Here's how the part is built. I have some questions about the finished solid (model axes, mm). Give positions to 0.01 mm unless a question says otherwise; leave off trailing zeros. Write each loop counter-clockwise with the first axis right and the second up, starting at its lowest first coordinate (ties: lowest second). Pieces come first, ordered by that corner, then holes. Notation, with made-up numbers: (49.5, 33) - (93.5, 33) arc R6 ccw to (93.5, 42) - close; hole circle Ø2 at (-26, -9.5). An arc over 180 degrees is marked (long way). Use a Markdown table: item, result.
Autodesk Inventor part; units mm, degrees
ref_plane "YZ Plane" through (0, 0, 0) normal (1, 0, 0) x (0, 1, 0)
ref_plane "XZ Plane" through (0, 0, 0) normal (0, 1, 0) x (-1, 0, 0)
ref_plane "XY Plane" through (0, 0, 0) normal (0, 0, 1) x (1, 0, 0)
sketch "スケッチ1" plane through (0, 0, 0) normal (0, 0, 1) x (1, 0, 0)
  circle A0 centre (104.0735, 2) radius 6.025
  arc A1 (100.4168, -2.7885) -> (70.6822, 5.0468) centre (76.1402, -34.5791) ccw
  line L0 (69.7806, -5) -> (104.0735, 2) construction
  circle A2 centre (69.7806, -5) radius 5 construction
  arc A3 (102.7574, -3.8795) -> (72.4739, -9.2126) centre (94.0202, -42.9136) ccw construction
  circle A4 centre (75.3506, 22) radius 5 construction
  circle A5 centre (70, 10) radius 1.5
  circle A6 centre (70, 10) radius 5
  arc A7 (109.4834, 4.652) -> (75.6055, 26.9935) centre (73.5667, -12.9545) ccw construction
  arc A8 (108.1244, 6.4599) -> (68.3957, 14.7356) centre (81.2303, -23.1494) ccw
  arc A9 (105.8851, 7.7462) -> (66.341, -1.371) centre (93.8576, -30.4027) ccw construction
  line L1 (70, 10) -> (104.0735, 2) construction
  circle A10 centre (82.0403, 11.2819) radius 1.5
  line L2 (48.483, 55.1333) -> (82.5564, 47.1333) construction
  line L3 (82.5564, 47.1333) -> (53.8336, 67.1333) construction
  line L4 (82.5564, 47.1333) -> (48.2636, 40.1333) construction
  circle A11 centre (53.8336, 67.1333) radius 5 construction
  circle A12 centre (48.2636, 40.1333) radius 5 construction
  circle A13 centre (48.483, 55.1333) radius 5
  circle A14 centre (82.5564, 47.1333) radius 1.5
  circle A15 centre (82.5564, 47.1333) radius 5
  circle A16 centre (48.483, 55.1333) radius 1.5
  arc A17 (77.6092, 46.4087) -> (54.8703, 62.242) centre (58.8098, 43.6549) ccw construction
  arc A18 (78.225, 44.6356) -> (51.2502, 50.9689) centre (61.7656, 35.1441) ccw
  arc A19 (79.6686, 43.0516) -> (52.5201, 37.51) centre (68.6948, 27.5411) ccw construction
  arc A20 (85.2716, 51.3319) -> (44.1201, 42.9319) centre (68.9807, 26.1405) ccw construction
  arc A21 (86.7799, 49.8095) -> (45.8918, 59.4095) centre (61.4389, 33.7524) ccw
  arc A22 (87.4691, 48.0636) -> (53.0017, 72.0636) centre (57.993, 42.4818) ccw construction
  circle A23 centre (82.5564, 47.1333) radius 4
  point P0 (0, 0)
  point P1 (0, 0)
  dimension "d0" = 40
  dimension "d1" = 10
  dimension "d2" = 40
  dimension "d3" = 10
  dimension "d4" = 10
  dimension "d5" = 3
  dimension "d6" = 19
  dimension "d7" = 30
  dimension "d8" = 3
  dimension "d9" = 8
extrude "押し出し1" add sketch "スケッチ1" along normal blind 3 contours A13 | A13 A21 A15 A18 | A15
properties part number "heikou平行" material "アルミニウム 2014-T4"
Item 1: If we section it at C-C, the plane y = 45.5: Write out the boundary of the cut face in (x, z).
Values:
| item | result |
|---|---|
| outline | (77.7, 0) - (78.91, 0) - (78.91, 3) - (77.7, 3) - close; (86.21, 0) - (87.28, 0) - (87.28, 3) - (86.21, 3) - close |
Item 2: Thinking about a two-plate mould opening in Y: for faces 1 (the cylindrical face through (49.869, 55.708, 1.479)), 2 (the cylindrical face through (65.9, 53.69, 1.48)), 3 (the cylindrical face through (67.98, 63.03, 1.48)), which applies, +Y half, -Y half, draft (parallel to the pull), parting line (faces both ways), or undercut?
Values:
| item | result |
|---|---|
| face 1 | undercut |
| face 2 | -Y half |
| face 3 | +Y half |
Item 3: If we section it at A-A, the plane x = 81.5: Write out the boundary of the cut face in (y, z), plus the area to 3 significant figures.
Values:
| item | result |
|---|---|
| outline | (42.25, 0) - (43.28, 0) - (43.28, 3) - (42.25, 3) - close; (50.99, 0) - (56.06, 0) - (56.06, 3) - (50.99, 3) - close |
| area | 18.3 mm2 |
Item 4: I need wall thicknesses on line 1 along X through (y, z) = (55.25, 1.5); line 2 along X through (y, z) = (56, 2.7); line 3 along Y through (x, z) = (79, 1.2). Which ranges of each line are inside material? Lowest first, please. Write a range as [from, to].
Values:
| item | result |
|---|---|
| line 1 | x = [43.48, 46.99], [49.98, 82.36] |
| line 2 | x = [43.56, 47.26], [49.71, 81.56] |
| line 3 | y = [43.62, 45.3], [48.96, 58.08] |
Item 5: If we section it at B-B, the plane z = 0.65: Write out the boundary of the cut face in (x, y) (1 decimal).
Values:
| item | result |
|---|---|
| outline | (45.9, 59.4) arc R5 ccw (long way) to (51.3, 51) arc R19 cw to (78.2, 44.6) arc R5 ccw (long way) to (86.8, 49.8) arc R30 ccw to start; hole circle Ø3 at (48.5, 55.1); hole circle Ø8 at (82.6, 47.1) |
Item 6: Will these pins go through, and if not, where does the flat tip stop? pin 1 Ø1 at (x, z) = (60, 1) entering from -Y; pin 2 Ø4 at (x, y) = (48.48, 55.13) entering from +Z; pin 3 Ø1.5 at (x, z) = (69, 2.5) entering from -Y; pin 4 Ø1.5 at (y, z) = (61, 1.5) entering from -X.
Values:
| item | result |
|---|---|
| pin 1 | stops at y = 54.01 |
| pin 2 | stops at z = 3 |
| pin 3 | stops at y = 52.39 |
| pin 4 | stops at x = 47.37 |
Item 7: If we section it at D-D, the plane y = 61.25: Write out the boundary of the cut face in (x, z), plus the area to 3 significant figures.
Values:
| item | result |
|---|---|
| outline | (49.44, 0) - (73.43, 0) - (73.43, 3) - (49.44, 3) - close |
| area | 72.0 mm2 |
